Geometry check sheet. Reference: drawing and pictorial views, mm from the part's lowest x, y, z. Round coordinates to 2 decimals unless told otherwise and drop trailing zeros. Write each loop counter-clockwise with the first axis right and the second up, starting at its lowest first coordinate (ties: lowest second). Pieces come first, ordered by that corner, then holes. Notation, with made-up numbers: M 44,63.25 L 81,63.25 A21 ccw 81,95.25 Z; hole C 47.5,-22 d4. An arc over 180 degrees is marked long. Answer in a Markdown table with one row per item. Add a question column.
1. Go/stop test with a flat-tipped pin: pin 1 Ø0.9 at (x, y) = (3, 3) entering from +Z. Record where the tip stops, or that it passes through.
2. Sectioned sample at A-A on y = 37. Record the cut outline in (x, z), plus the area to 3 significant figures.
3. Material ranges on probe 1 along X at (y, z) = (37, 5.25); probe 2 along X at (y, z) = (36.5, 1.5), recorded low to high.
4. Sectioned sample at B-B on z = 6.5. Record the cut outline in (x, y).
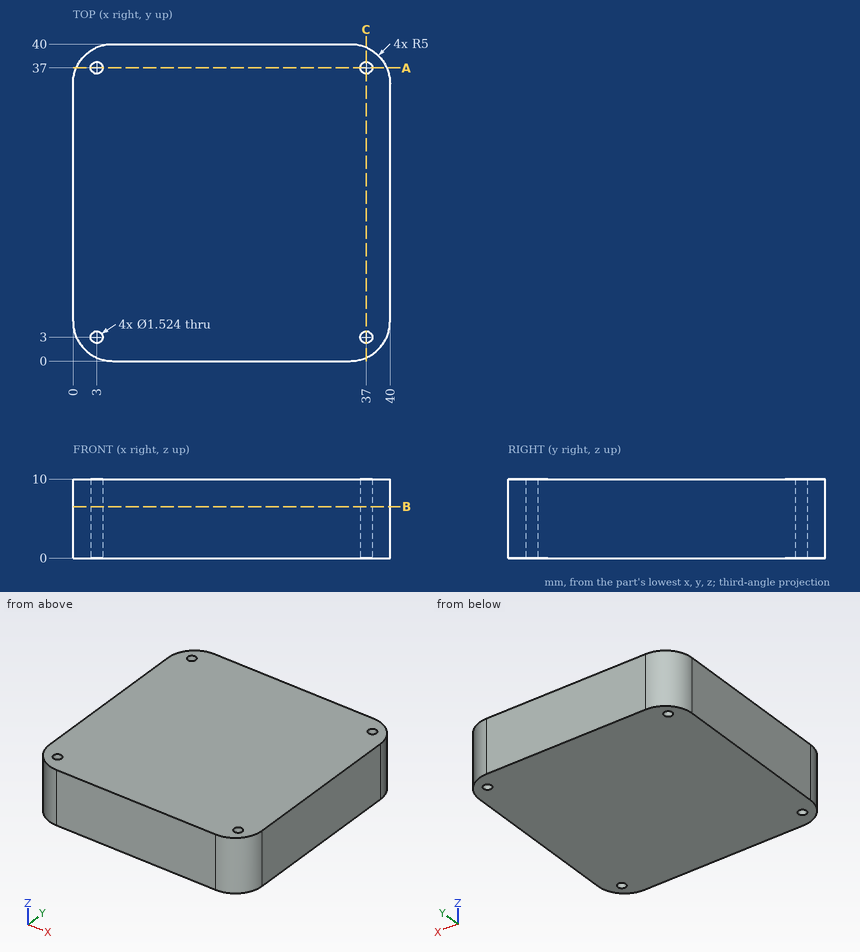
Geometry check:
| question | item | result |
|---|---|---|
| 1 | pin 1 | passes through |
| 2 | outline | M 0.42,0 L 2.24,0 L 2.24,10 L 0.42,10 Z; M 3.76,0 L 36.24,0 L 36.24,10 L 3.76,10 Z; M 37.76,0 L 39.58,0 L 39.58,10 L 37.76,10 Z |
| 2 | area | 361 mm2 |
| 3 | probe 1 | x = 0.42 to 2.24, 3.76 to 36.24, 37.76 to 39.58 |
| 3 | probe 2 | x = 0.23 to 2.42, 3.58 to 36.42, 37.58 to 39.77 |
| 4 | outline | M 0,5 A5 ccw 5,0 L 35,0 A5 ccw 40,5 L 40,35 A5 ccw 35,40 L 5,40 A5 ccw 0,35 Z; hole C 3,3 d1.52; hole C 3,37 d1.52; hole C 37,3 d1.52; hole C 37,37 d1.52 |
